For this review, use the dimensioned drawing (mm, ordinates from the lowest corner) and the shaded views. A direction names the side the tool comes from. Round coordinates to 2 decimals unless told otherwise and drop trailing zeros. Loops run counter-clockwise (first coordinate to the right, second up) from the corner with the lowest first, then second, coordinate; pieces in that order, holes last. Notation, with made-up numbers: (45.25, -14) -> (98.25, -14) arc R24 cw to (98.25, 1) -> close; hole circle Ø10 at (87.5, -7.75). An arc over 180 degrees is marked (long way). Use one line per item in the form item = value. Start each with the question number.
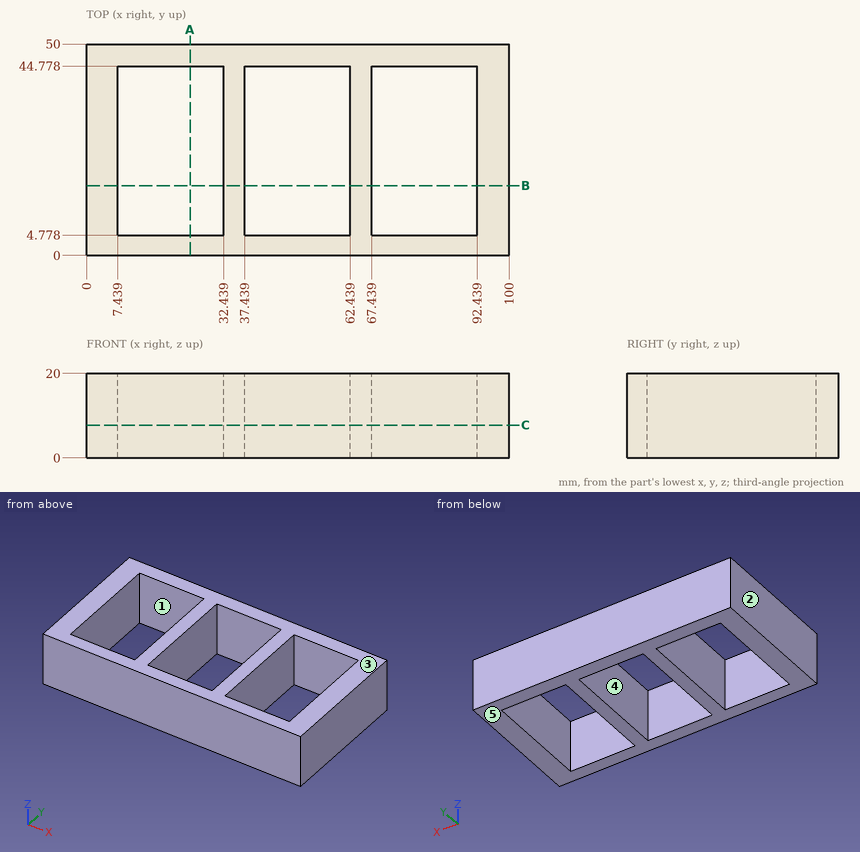
Item 1: Take a section at A-A on x = 24.5. Give the boundary of the cut face in (y, z).
Item 2: Wall thickness on line 1 (X direction, y = 30, z = 18); line 2 (Y direction, x = 8, z = 18.25): over which ranges is each line inside the solid? List them lowest first.
Item 3: Take a section at C-C on z = 7.75. Give the boundary of the cut face in (x, y).
Item 4: Take a section at B-B on y = 16.5. Give the boundary of the cut face in (x, z).
Item 5: Draft analysis for pull direction X (two halves, no side actions). For the marked faces 1, 2 and 3, state which applies: +X half, -X half, draft (parallel to the pull), parting line (faces both ways), or undercut.
Item 6: Machinability: for the marked faces 4 and 5, which of the approach directions +Z, -Z, +X, -X, +Y, -Y give a long, thin tool a straight path to every point of the face, cutting with its end or side? Answer none if there is none.
Results:
q1.outline = (0, 0) -> (4.78, 0) -> (4.78, 20) -> (0, 20) -> close; (44.78, 0) -> (50, 0) -> (50, 20) -> (44.78, 20) -> close
q2.line_1 = 0 to 7.44, 32.44 to 37.44, 62.44 to 67.44, 92.44 to 100
q2.line_2 = 0 to 4.78, 44.78 to 50
q3.outline = (0, 0) -> (100, 0) -> (100, 50) -> (0, 50) -> close; hole (7.44, 4.78) -> (32.44, 4.78) -> (32.44, 44.78) -> (7.44, 44.78) -> close; hole (37.44, 4.78) -> (62.44, 4.78) -> (62.44, 44.78) -> (37.44, 44.78) -> close; hole (67.44, 4.78) -> (92.44, 4.78) -> (92.44, 44.78) -> (67.44, 44.78) -> close
q4.outline = (0, 0) -> (7.44, 0) -> (7.44, 20) -> (0, 20) -> close; (32.44, 0) -> (37.44, 0) -> (37.44, 20) -> (32.44, 20) -> close; (62.44, 0) -> (67.44, 0) -> (67.44, 20) -> (62.44, 20) -> close; (92.44, 0) -> (100, 0) -> (100, 20) -> (92.44, 20) -> close
q5.face_1 = undercut
q5.face_2 = -X half
q5.face_3 = draft
q6.face_4 = +Z, -Z
q6.face_5 = -Z, +X, -X, +Y, -Y
